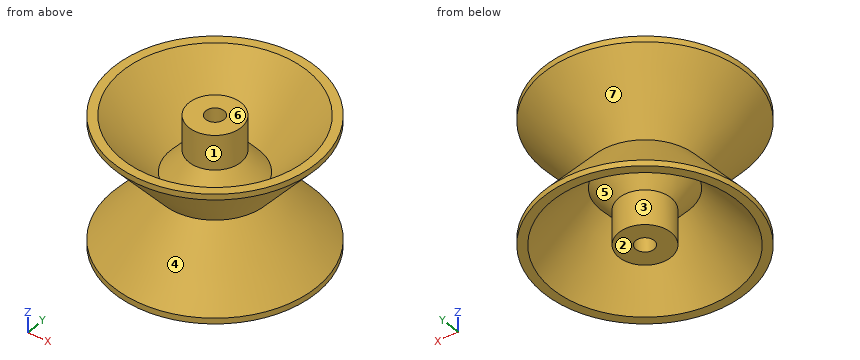
from build123d import *


with BuildPart() as part:
    # Sketch1 → Revolve1 (revolve)
    with BuildSketch(Plane(origin=(0, 0, 0), x_dir=(1, 0, 0), z_dir=(0, 1, 0))):
        with BuildLine():
            Line((3.175, 0), (3.175, 5))
            ThreePointArc((3.175, 5), (4.529564638, 7.346174775), (5, 10.014146291))
            Line((5, 10.014146291), (5, 34.985853709))
            ThreePointArc((5, 34.985853709), (4.529564638, 37.653825225), (3.175, 40))
            Line((3.175, 40), (3.175, 45))
            Line((3.175, 45), (9, 45))
            Line((9, 45), (9, 32.985593407))
            Line((9, 32.985593407), (15.45935793, 25.287630389))
            Line((15.45935793, 25.287630389), (32, 45))
            Line((32, 45), (35, 45))
            Line((35, 45), (35, 43))
            Line((35, 43), (17.798457561, 22.5))
            Line((17.798457561, 22.5), (35, 2))
            Line((35, 2), (35, 0))
            Line((35, 0), (32, 0))
            Line((32, 0), (15.45935793, 19.712369611))
            Line((15.45935793, 19.712369611), (9, 12.014406593))
            Line((9, 12.014406593), (9, 0))
            Line((9, 0), (3.175, 0))
        make_face()
    revolve(axis=Axis((0, 0, 0), (0, 0, -1)))


solid = part.part
The model under review builds one solid part; all positions refer to its coordinate system, in mm. Face numbers are marked on the shaded views. A direction names the side the tool comes from. Coordinates: 2 decimals unless noted, no trailing zeros. Loops run counter-clockwise (first coordinate to the right, second up) from the corner with the lowest first, then second, coordinate; pieces in that order, holes last. Notation, with made-up numbers: (14, -36.5) -> (63, -36.5) arc R21 ccw to (63, -18.5) -> close; hole circle Ø5 at (38.25, 24). An arc over 180 degrees is marked (long way). Use a Markdown table: item, result. Add a question column.
1. Add section B-B on z = -9. Give the number of separate pieces and of enclosed holes in the cut face, plus the area to 3 significant figures.
2. Clearance check with flat-ended pins moving along their axes: pin 1 Ø4 at (x, z) = (-10.5, -36) entering from -Y; pin 2 Ø1 at (x, z) = (7, -29.5) entering from -Y; pin 3 Ø6 at (x, z) = (12.5, -5.5) entering from +Y; pin 4 Ø6 at (y, z) = (-28, -29.5) entering from +X. State where each tip first meets the part, or that it passes through.
3. To check wall thickness, follow line 1 (X direction, y = 8, z = -2); line 2 (Y direction, x = 0, z = -3.45) (3 decimals); line 3 (X direction, y = 0, z = -41) (3 decimals). State the ranges of each line that lie inside material, in increasing order.
4. Draft analysis for pull direction Y (two halves, no side actions). For the marked faces 5, 6 and 7, state which applies: pulls with the +Y half, pulls with the -Y half, needs draft (parallel to the pull), parting line crosses it, or undercut.
5. Add section A-A on z = -28. Write out the cut boundary in (x, y).
6. Machinability: for the marked faces 1, 2, 3 and 4, which of the approach directions +Z, -Z, +X, -X, +Y, -Y give a long, thin tool a straight path to every point of the face, cutting with its end or side? Answer none if there is none.
Returned:
| question | item | result |
|---|---|---|
| 1 | separate pieces | 2 |
| 1 | enclosed holes | 2 |
| 1 | area | 965 mm² |
| 2 | pin 1 | stops at y = -29.09 |
| 2 | pin 2 | stops at y = -23.08 |
| 2 | pin 3 | stops at y = 32.46 |
| 2 | pin 4 | passes through |
| 3 | line 1 | x = -34.07 to -29.25, -4.12 to 4.12, 29.25 to 34.07 |
| 3 | line 2 | y = -33.783 to -29.105, -9 to -3.175, 3.175 to 9, 29.105 to 33.783 |
| 3 | line 3 | x = -33.322 to -28.644, -9 to -3.175, 3.175 to 9, 28.644 to 33.322 |
| 4 | face 5 | undercut |
| 4 | face 6 | needs draft |
| 4 | face 7 | parting line crosses it |
| 5 | outline | circle Ø44.83 at (0, 0); circle Ø26.37 at (0, 0); hole circle Ø35.47 at (0, 0); hole circle Ø10 at (0, 0) |
| 6 | face 1 | +Z |
| 6 | face 2 | -Z, +X, -X, +Y, -Y |
| 6 | face 3 | -Z |
| 6 | face 4 | none |
